Verification items for the finished model (mm, model axes). Face numbers are marked on the shaded views. A direction names the side the tool comes from. Round coordinates to 2 decimals unless told otherwise and drop trailing zeros. Write each loop counter-clockwise with the first axis right and the second up, starting at its lowest first coordinate (ties: lowest second). Pieces come first, ordered by that corner, then holes. Notation, with made-up numbers: M 81,-7.5 L 114,-7.5 A24 cw 114,19.5 Z; hole C 76.5,7 d8. An arc over 180 degrees is marked long. Use a Markdown table: item, result. Add a question column.
from build123d import *

# Parameters (mm, degrees)
F1_W     = 95.06
F1_H     = 73.2
F2_DEPTH = 22
F3_W     = 85.06
F3_H     = 65.4996002525
F4_DEPTH = 17
F5_W     = 13
F5_H     = 12
F6_DEPTH = 5
F5_W_2   = 10
F7_DEPTH = 5


with BuildPart() as f2:
    # F1 (on Top) → F2 (new body)
    with BuildSketch(Plane.XY):
        with Locations((-6.269495101, -12.3295125008)):
            Rectangle(F1_W, F1_H)
    extrude(amount=F2_DEPTH)

    # F3 (on face) → F4 (cut)
    with BuildSketch(Plane.XY.offset(22)):
        with Locations((-6.269495101, -12.3295125008)):
            Rectangle(F3_W, F3_H)
    extrude(amount=-F4_DEPTH, mode=Mode.SUBTRACT)

    # F5 (on face) → F6 (cut)
    with BuildSketch(Plane(origin=(-53.799495101, 0, 0), x_dir=(0, -1, 0), z_dir=(-1, 0, 0))):
        with Locations((1.2295125008, 12.5)):
            Rectangle(F5_W, F5_H)
    extrude(amount=-F6_DEPTH, mode=Mode.SUBTRACT)

    # F5 (on face) → F7 (cut)
    with BuildSketch(Plane(origin=(-53.799495101, 0, 0), x_dir=(0, -1, 0), z_dir=(-1, 0, 0))):
        with Locations((31.1295125008, 12.5)):
            Rectangle(F5_W_2, F5_H)
    extrude(amount=-F7_DEPTH, mode=Mode.SUBTRACT)


solid = f2.part
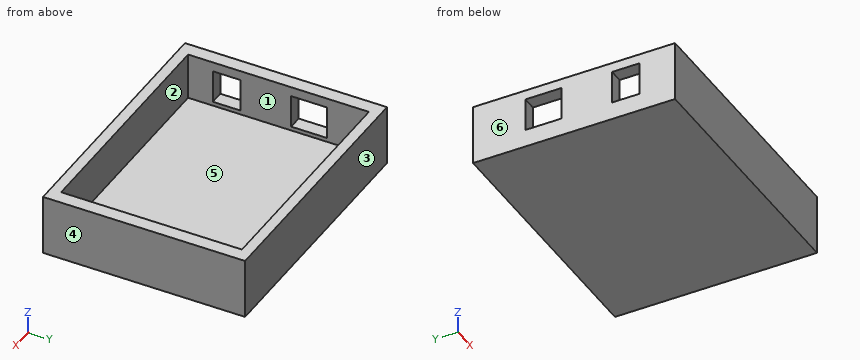
1. Cross-section at B-B on z = 19.75. Enter the section's corners in (x, y), plus the area to 3 significant figures.
2. Scan lines: line 1 along Y through (x, z) = (2.5, 6.5); line 2 along X through (y, z) = (-37, 11); line 3 along Z through (x, y) = (-13.5, 18). Record each from-to range of solid material in increasing order. Write a range as from..to.
3. Depth check by flat-ended pin: pin 1 Ø3 at (x, y) = (20.5, -23.5) entering from +Z. Enter the tip coordinate at first touch or a pass-through.
4. Cross-section at D-D on x = 25. Enter the section's corners in (y, z).
5. Release check for a two-part mould opening along X. For the marked faces 1, 2, 3 and 4 record: +X half, -X half, draft (parallel to the pull), parting line (faces both ways), or undercut.
6. Cross-section at A-A on y = -1. Enter the section's corners in (x, z), plus the area to 3 significant figures.
7. Access from +Z, -Z, +X, -X, +Y, -Y to the whole of each face (thin tool, end or side, straight path). Record for the marked faces 5 and 6.
8. Cross-section at C-C on z = 8. Enter the section's corners in (x, y), plus the area to 3 significant figures.
Answer:
| question | item | result |
|---|---|---|
| 1 | outline | M -53.8,-48.93 L 41.26,-48.93 L 41.26,24.27 L -53.8,24.27 Z; hole M -48.8,-45.08 L 36.26,-45.08 L 36.26,20.42 L -48.8,20.42 Z |
| 1 | area | 1,390 mm^2 |
| 2 | line 1 | y = -48.93..-45.08, 20.42..24.27 |
| 2 | line 2 | x = -53.8..-48.8, 36.26..41.26 |
| 2 | line 3 | z = 0..5 |
| 3 | pin 1 | stops at z = 5 |
| 4 | outline | M -48.93,0 L 24.27,0 L 24.27,22 L 20.42,22 L 20.42,5 L -45.08,5 L -45.08,22 L -48.93,22 Z |
| 5 | face 1 | undercut |
| 5 | face 2 | undercut |
| 5 | face 3 | draft |
| 5 | face 4 | +X half |
| 6 | outline | M -53.8,0 L 41.26,0 L 41.26,22 L 36.26,22 L 36.26,5 L -48.8,5 L -48.8,6.5 L -53.8,6.5 Z; M -53.8,18.5 L -48.8,18.5 L -48.8,22 L -53.8,22 Z |
| 6 | area | 585 mm^2 |
| 7 | face 5 | +Z |
| 7 | face 6 | +Z, -Z, -X, +Y, -Y |
| 8 | outline | M -53.8,-48.93 L 41.26,-48.93 L 41.26,24.27 L -53.8,24.27 L -53.8,5.27 L -48.8,5.27 L -48.8,20.42 L 36.26,20.42 L 36.26,-45.08 L -48.8,-45.08 L -48.8,-36.13 L -53.8,-36.13 Z; M -53.8,-26.13 L -48.8,-26.13 L -48.8,-7.73 L -53.8,-7.73 Z |
| 8 | area | 1,270 mm^2 |
